Input: dimensioned drawing with shaded views. Units: mm. Origin: part minimum x, y, z. Coordinates: 2 decimals unless noted, no trailing zeros. Loops run counter-clockwise (first coordinate to the right, second up) from the corner with the lowest first, then second, coordinate; pieces in that order, holes last. Notation, with made-up numbers: (76.5, 80.5) - (108.5, 80.5) arc R16 ccw to (108.5, 91.5) - close; hole circle Ø5 at (-2, 44.5). An arc over 180 degrees is marked (long way). Put each result on its own line as item: value. Start each with the question number.
1) Draft query along X for the marked faces 1, 2 and 3. Return one class per face: +X half, -X half, draft (parallel to the pull), parting line (faces both ways), or undercut.
2) Section A-A on x = 23. Output: boundary loops of the cut face in (y, z).
3) Material intervals for line 1 along Y through (x, z) = (23, 13.1); line 2 along Z through (x, y) = (25, 11.5); line 3 along Y through (x, z) = (27, 14), sorted ascending. Write a range as from..to.
4) Section D-D on z = 5.5. Output: boundary loops of the cut face in (x, y), and give its area (3 significant figures).
5) Contact query for flat-ended pins moving along their axis: pin 1 Ø5 at (x, y) = (26, 36) entering from +Z; pin 2 Ø5 at (x, z) = (20.5, 4.5) entering from +Y; pin 3 Ø1.5 at (x, z) = (8.5, 13.5) entering from +Y. Output: stop coordinate, or through.
6) Section C-C on z = 13.5. Output: boundary loops of the cut face in (x, y), and give its area (3 significant figures).
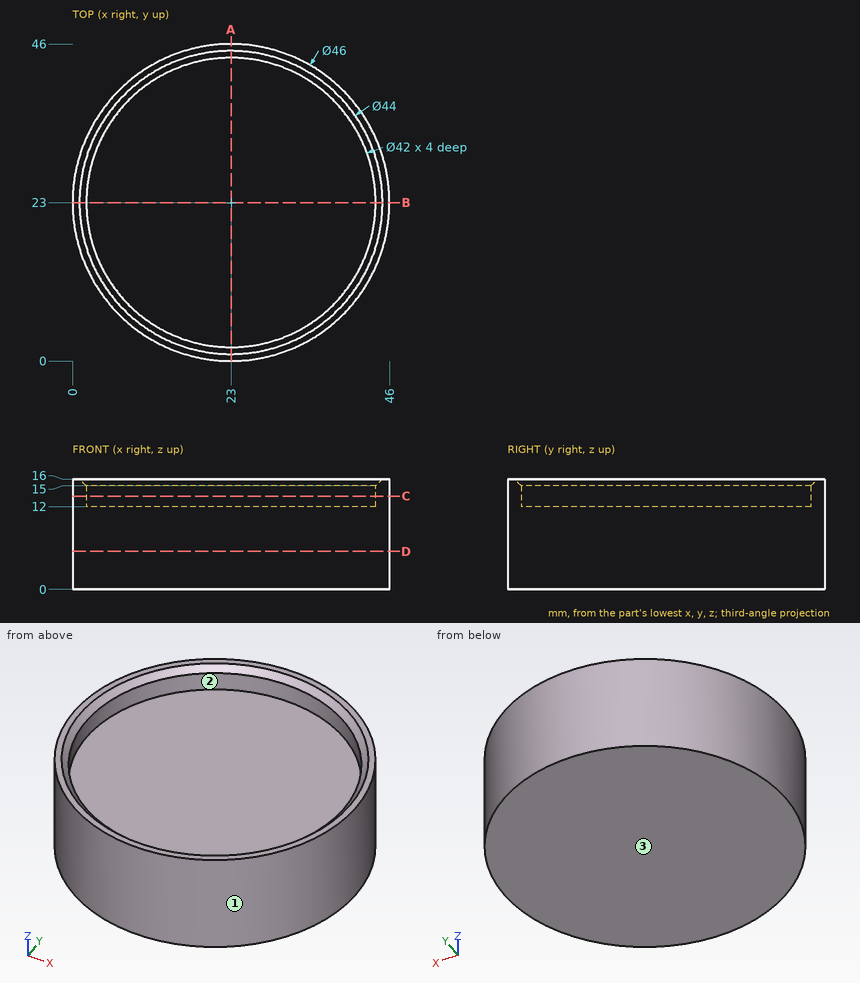
Answer block:
1. face 1: parting line
1. face 2: undercut
1. face 3: draft
2. outline: (0, 0) - (46, 0) - (46, 16) - (45, 16) - (44, 15) - (44, 12) - (2, 12) - (2, 15) - (1, 16) - (0, 16) - close
3. line 1: y = 0..2, 44..46
3. line 2: z = 0..12
3. line 3: y = 0.35..2.38, 43.62..45.65
4. outline: circle Ø46 at (23, 23)
4. area: 1,660 mm²
5. pin 1: stops at z = 12
5. pin 2: stops at y = 46
5. pin 3: stops at y = 41.44
6. outline: circle Ø46 at (23, 23); hole circle Ø42 at (23, 23)
6. area: 276 mm²
